```python
from build123d import *

# Parameters (mm, degrees)
ESQUISSE1_W      = 10
ESQUISSE1_H      = 10
ESQUISSE1_R      = 2
EXTRUSION1_DEPTH = 1
ESQUISSE2_W      = 1
ESQUISSE2_H      = 10
EXTRUSION2_DEPTH = 9
EXTRUSION3_REACH = 12
ESQUISSE3_R      = 2


with BuildPart() as part:
    # Esquisse1 → Extrusion1 (new body)
    with BuildSketch(Plane(origin=(0, 0, 0), x_dir=(1, 0, 0), z_dir=(0, 1, 0))):
        with Locations((5, 5)):
            Rectangle(ESQUISSE1_W, ESQUISSE1_H)
        with Locations((5, 5)):
            Circle(ESQUISSE1_R, mode=Mode.SUBTRACT)
    extrude(amount=EXTRUSION1_DEPTH)

    # Esquisse2 → Extrusion2 (add)
    with BuildSketch(Plane(origin=(0, 1, 0), x_dir=(1, 0, 0), z_dir=(0, 1, 0))):
        with Locations((9.5, 5)):
            Rectangle(ESQUISSE2_W, ESQUISSE2_H)
    extrude(amount=EXTRUSION2_DEPTH)

    # Esquisse3 → Extrusion3 (cut, up to next)
    with BuildSketch(Plane(origin=(10, 0, 0), x_dir=(0, 0, -1), z_dir=(1, 0, 0)), mode=Mode.PRIVATE) as extrusion3_sk1:
        with Locations((5, 5)):
            Circle(ESQUISSE3_R)
    extrusion3_tool1 = extrude(extrusion3_sk1.sketch, amount=-EXTRUSION3_REACH, mode=Mode.PRIVATE) & part.part
    add(extrusion3_tool1.solids().sort_by_distance((10, 5, -5))[0], mode=Mode.SUBTRACT)


solid = part.part
```
Check sheet for the modelled part. Datum: model origin and axes. Units: mm. A direction names the side the tool comes from. Round coordinates to 2 decimals unless told otherwise and drop trailing zeros. Write each loop counter-clockwise with the first axis right and the second up, starting at its lowest first coordinate (ties: lowest second). Pieces come first, ordered by that corner, then holes. Notation, with made-up numbers: (40.25, 21) -> (81.25, 21) arc R28 cw to (81.25, 51) -> close; hole circle Ø7 at (29, 87). An arc over 180 degrees is marked (long way). Put each result on its own line as item: value.
(1) Sectioned sample at B-B (x = 5). Enter the section's corners in (y, z), plus the area to 3 significant figures.
Values found:
outline: (0, -10) -> (1, -10) -> (1, -7) -> (0, -7) -> close; (0, -3) -> (1, -3) -> (1, 0) -> (0, 0) -> close
area: 6.00 mm^2
(2) Tool access check on faces 1 (the face through (9, 7.4, -4.9)), 2 (the face through (10, 4.9, -7.2)). Record the directions out of +Z, -Z, +X, -X, +Y, -Y that give a thin tool (end or side, any length) a straight path to the whole face; none if there is none.
Values found:
face 1: +Z, -Z, -X, +Y
face 2: +Z, -Z, +X, +Y, -Y
(3) Go/stop test with flat-tipped pins: pin 1 Ø4.5 at (y, z) = (5, -5) entering from +X; pin 2 Ø2 at (x, y) = (7.5, 6.5) entering from +Z; pin 3 Ø3 at (y, z) = (5.5, -8.5) entering from -X. Record where each tip stops, or that it passes through.
Values found:
pin 1: stops at x = 10
pin 2: passes through
pin 3: stops at x = 9
(4) Sectioned sample at A-A (y = 5). Enter the section's corners in (x, z), plus the area to 3 significant figures.
Values found:
outline: (9, -10) -> (10, -10) -> (10, -7) -> (9, -7) -> close; (9, -3) -> (10, -3) -> (10, 0) -> (9, 0) -> close
area: 6.00 mm^2
(5) Sectioned sample at C-C (z = -5). Enter the section's corners in (x, y), plus the area to 3 significant figures.
Values found:
outline: (0, 0) -> (3, 0) -> (3, 1) -> (0, 1) -> close; (7, 0) -> (10, 0) -> (10, 3) -> (9, 3) -> (9, 1) -> (7, 1) -> close; (9, 7) -> (10, 7) -> (10, 10) -> (9, 10) -> close
area: 11.0 mm^2
(6) Mould release check, pull along Z, two halves, no side actions. Record for faces 3 (the face through (9.507, 5.088, -3.002)), 4 (the face through (0, 0.5, -4.9)): released by +Z, released by -Z, zero draft, split by the parting line, or undercut.
Values found:
face 3: undercut
face 4: zero draft
(7) Sectioned sample at D-D (x = 2.75). Enter the section's corners in (y, z), plus the area to 3 significant figures.
Values found:
outline: (0, -10) -> (1, -10) -> (1, 0) -> (0, 0) -> close
area: 10.0 mm^2
(8) Material ranges on line 1 (Y direction, x = 9.3, z = -5); line 2 (X direction, y = 7, z = -8.75), recorded low to high.
Values found:
line 1: y = 0 to 3, 7 to 10
line 2: x = 9 to 10
